Here's how the part is built. I have some questions about the finished solid (model axes, mm). Round coordinates to 2 decimals unless told otherwise and drop trailing zeros. Write each loop counter-clockwise with the first axis right and the second up, starting at its lowest first coordinate (ties: lowest second). Pieces come first, ordered by that corner, then holes. Notation, with made-up numbers: M 89.5,0 L 93.5,0 A16 ccw 93.5,8 Z; hole C 27,63.25 d3. An arc over 180 degrees is marked long. Use one line per item in the form item = value. Start each with the question number.
Q1. I need wall thicknesses on line 1 along X through (y, z) = (1.45, -26); line 2 along Z through (x, y) = (-3, 1.45); line 3 along Z through (x, y) = (-6, 2.25). Which ranges of each line are inside material? Lowest first, please. Write a range as from..to.
Q2. I'm going to push flat-ended pins straight in: pin 1 Ø15 at (x, z) = (0, -9) entering from -Y; pin 2 Ø1.5 at (y, z) = (1, 21) entering from +X; pin 3 Ø2.5 at (x, z) = (0, 9) entering from +Y; pin 4 Ø6 at (x, z) = (-1.5, 7) entering from +Y. Where does each tip first touch, or does it pass through?
Q3. I want a section at D-D on x = -30.5. List the corners of the cut face in (y, z) for me, and give its area (3 significant figures).
Q4. I want a section at B-B on z = -9. List the corners of the cut face in (x, y) for me.
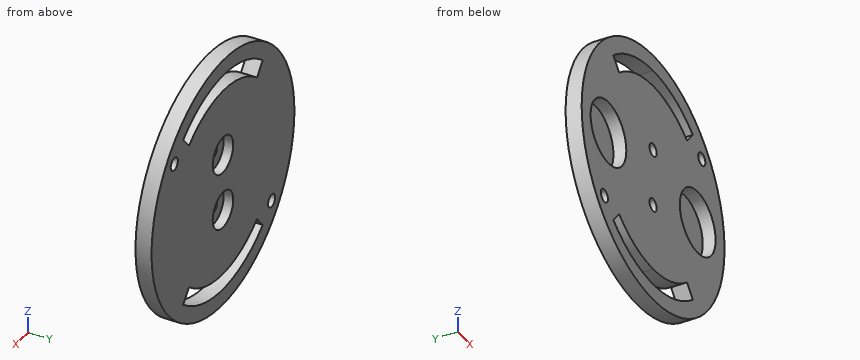
Autodesk Inventor part; units mm, degrees
ref_plane "Work Plane1" through (0, 0, 32.5) normal (1, 0, 0) x (0, 0, -1)
ref_plane "YZ Plane" through (0, 0, 0) normal (1, 0, 0) x (0, 1, 0)
ref_plane "XZ Plane" through (0, 0, 0) normal (0, 1, 0) x (-1, 0, 0)
sketch "Sketch1" plane through (0, 0, 0) normal (0, 1, 0) x (-1, 0, 0)
  circle A0 centre (0, 0) radius 40
  dimension "d0" = 80
sketch "Sketch1 outline for Extrusion1" plane through (0, 0, 0) normal (0, 1, 0) x (-1, 0, 0)
  circle A0 centre (0, 0) radius 40
extrude "Extrusion1" add sketch "Sketch1 outline for Extrusion1" along normal blind 5
sketch "Sketch3" plane through (0, 5, 0) normal (0, 1, 0) x (1, 0, 0)
  line L0 (0, 0) -> (-5, 0)
  line L1 (0, 0) -> (5, 0)
  line L2 (0, 0) -> (0, -9)
  line L3 (0, 0) -> (0, 9)
  circle A0 centre (0, 9) radius 2
  circle A1 centre (0, -9) radius 2
  dimension "d63" = 9
  dimension "d64" = 9
  dimension "d65" = 4
  dimension "d66" = 4
sketch "Sketch3 outline for Extrusion3" plane through (0, 5, 0) normal (0, 1, 0) x (1, 0, 0)
  circle A0 centre (0, 9) radius 2
  circle A1 centre (0, -9) radius 2
extrude "Extrusion3" cut sketch "Sketch3 outline for Extrusion3" against normal up to surface (5 mm away)
sketch "Sketch6" plane through (0, 0, 0) normal (0, -1, 0) x (1, 0, 0)
  line L0 (0, 0) -> (-25, 0)
  line L1 (0, 0) -> (25, 0)
  circle A0 centre (25, 0) radius 10
  circle A1 centre (-25, 0) radius 10
  dimension "d18" = 25
  dimension "d19" = 25
  dimension "d20" = 20
  dimension "d21" = 20
sketch "Sketch6 outline for Extrusion5" plane through (0, 0, 0) normal (0, -1, 0) x (1, 0, 0)
  circle A0 centre (25, 0) radius 10
  circle A1 centre (-25, 0) radius 10
extrude "Extrusion5" cut sketch "Sketch6 outline for Extrusion5" against normal blind 4
sketch "Sketch8" plane through (0, 0, 0) normal (0, -1, 0) x (1, 0, 0)
  circle A0 centre (0, 0) radius 40
  line L0 (0, 40) -> (0, 35)
  line L1 (0, 35) -> (0, 30)
  line L2 (0, 30) -> (0, 27)
  circle A1 centre (0, 0) radius 35
  circle A2 centre (0, 0) radius 30
  line L3 (0, 27) -> (30, 27)
  line L4 (22.271057, 27) -> (19.056987, 23.169619)
  line L5 (22.271057, 27) -> (27.271264, 27) construction
  line L6 (-40, 0) -> (40, 0)
  line L7 (22.271057, -27) -> (19.056987, -23.169619)
  line L8 (0, -40) -> (0, -30)
  point P0 (0, -35)
  dimension "d46" = 5
  dimension "d47" = 5
  dimension "d48" = 3
  dimension "d49" = 130
sketch "Sketch8 outline for Extrusion7" plane through (0, 0, 0) normal (0, -1, 0) x (1, 0, 0)
  line L0 (0, -30) -> (0, -35)
  arc A0 (19.056987, -23.169619) -> (0, -30) centre (0, 0) cw
  line L1 (22.271057, -27) -> (19.056987, -23.169619)
  arc A1 (0, -35) -> (22.271057, -27) centre (0, 0) ccw
  arc A2 (22.271057, 27) -> (0, 35) centre (0, 0) ccw
  line L2 (19.056987, 23.169619) -> (22.271057, 27)
  arc A3 (0, 30) -> (19.056987, 23.169619) centre (0, 0) cw
  line L3 (0, 35) -> (0, 30)
extrude "Extrusion7" cut sketch "Sketch8 outline for Extrusion7" against normal up to surface (5 mm away)
ref_plane "Work Plane1" through (0, 0, 32.5) normal (1, 0, 0) x (0, 0, -1)
mirror "Mirror1" about plane through (0, 0, 32.5) normal (1, 0, 0) of "Extrusion7"
sketch "Sketch11" plane through (0, 5, 0) normal (0, 1, 0) x (1, 0, 0)
  circle A0 centre (0, -9) radius 2
  circle A1 centre (0, -9) radius 5.75
  circle A2 centre (0, 9) radius 2
  circle A3 centre (0, 9) radius 5.75
  point P0 (0, 0)
  dimension "d67" = 11.5
  dimension "d68" = 11.5
sketch "Sketch11 outline for Extrusion10" plane through (0, 5, 0) normal (0, 1, 0) x (1, 0, 0)
  circle A0 centre (0, 9) radius 5.75
  circle A1 centre (0, 9) radius 2
  circle A2 centre (0, -9) radius 5.75
  circle A3 centre (0, -9) radius 2
extrude "Extrusion10" cut sketch "Sketch11 outline for Extrusion10" against normal blind 3
sketch "Sketch12" plane through (0, 0, 0) normal (0, -1, 0) x (1, 0, 0)
  circle A0 centre (0, 0) radius 40
  line L0 (0, -40) -> (0, -35)
  arc A1 (-22.271057, -27) -> (22.271057, -27) centre (0, 0) ccw
  arc A2 (-19.056987, -23.169619) -> (19.056987, -23.169619) centre (0, 0) ccw
  circle A3 centre (-25, 0) radius 10
  line L1 (22.271057, 27) -> (22.271057, 22)
  line L2 (22.271057, 22) -> (27.271057, 22)
  circle A4 centre (27.271057, 22) radius 2
  line L3 (-22.271057, -27) -> (-22.271057, -22)
  line L4 (-22.271057, -22) -> (-27.271057, -22)
  circle A5 centre (-27.271057, -22) radius 2
  dimension "d71" = 5
  dimension "d72" = 5
  dimension "d73" = 4
  dimension "d74" = 5
  dimension "d75" = 5
  dimension "d76" = 4
sketch "Sketch12 outline for Extrusion11" plane through (0, 0, 0) normal (0, -1, 0) x (1, 0, 0)
  circle A0 centre (-27.271057, -22) radius 2
  circle A1 centre (27.271057, 22) radius 2
extrude "Extrusion11" cut sketch "Sketch12 outline for Extrusion11" against normal up to surface (5 mm away)
properties part number "Wrist_Arm"
Reported:
q1.line_1 = -30.4..-21.43, -14.97..14.97, 21.43..30.4
q1.line_2 = -39.89..-34.87, -29.85..29.85, 34.87..39.89
q1.line_3 = -39.55..-34.48, -29.39..29.39, 34.48..39.55
q2.pin_1 = 0
q2.pin_2 = 34.5
q2.pin_3 = through
q2.pin_4 = 2
q3.outline = M 0,-25.88 L 5,-25.88 L 5,25.88 L 0,25.88 L 0,8.35 L 4,8.35 L 4,-8.35 L 0,-8.35 Z
q3.area = 192 mm^2
q4.outline = M -38.97,0 L -29.36,0 L -29.36,4 L -20.64,4 L -20.64,0 L -2,0 L -2,2 L -5.75,2 L -5.75,5 L -38.97,5 Z; M 2,0 L 20.64,0 L 20.64,4 L 29.36,4 L 29.36,0 L 38.97,0 L 38.97,5 L 5.75,5 L 5.75,2 L 2,2 Z
